The listing builds one solid part. Answer for the finished solid, in the listing's coordinates (mm). A direction names the side the tool comes from. Coordinates: 2 decimals unless noted, no trailing zeros. Write each loop counter-clockwise with the first axis right and the second up, starting at its lowest first coordinate (ties: lowest second). Pieces come first, ordered by that corner, then holes. Notation, with made-up numbers: M -19.75,8 L 33.25,8 A17 cw 33.25,24 Z; hole C 47,36 d1. An arc over 180 degrees is marked long. Write item = value, one per line. Start each with the question number.
```python
from build123d import *

# Parameters (mm, degrees)
SKETCH_1_R          = 1
EXTRUDE_1_DEPTH     = 7
SKETCH_2_R          = 3.75
EXTRUDE_2_DEPTH     = 1
SKETCH_3_W          = 8.378804874
SKETCH_3_H          = 1
CUT_EXTRUDE_1_DEPTH = 0.5


with BuildPart() as part:
    # 草图1 → 拉伸1 (new body)
    with BuildSketch(Plane(origin=(0, 0, 0), x_dir=(1, 0, 0), z_dir=(0, 1, 0))):
        with Locations(Location((0, 0, 0), (0, 0, 270))):
            Circle(SKETCH_1_R)
    extrude(amount=EXTRUDE_1_DEPTH)

    # 草图2 → 拉伸2 (add)
    with BuildSketch(Plane(origin=(0, 7, 0), x_dir=(-1, 0, 0), z_dir=(0, 1, 0))):
        with Locations(Location((0, 0, 0), (0, 0, 90))):
            Circle(SKETCH_2_R)
    extrude(amount=EXTRUDE_2_DEPTH)

    # 草图3 → 切除-拉伸1 (cut)
    with BuildSketch(Plane(origin=(0, 8, 0), x_dir=(-1, 0, 0), z_dir=(0, 1, 0))):
        Rectangle(SKETCH_3_W, SKETCH_3_H)
    extrude(amount=-CUT_EXTRUDE_1_DEPTH, mode=Mode.SUBTRACT)


solid = part.part
```
1. The part is cut by section C-C, the plane y = 3.75. Write down the section's boundary in (x, z), and give its area (3 significant figures).
2. Straight lines are drawn through the part: L1, parallel to Y at x = 3, z = 1; L2, parallel to Z at x = -0.25, y = 4.25; L3, parallel to X at y = 0.5, z = -0.5. For each, find the intervals that lie inside material, in ascending order. Write a range as [from, to].
3. For a pull along Z with two mould halves and no side action, classify faces 1 (the face through (0, 7.5, 0)), 2 (the face through (0, 8, 2)), 3 (the face through (-1, 3, 0)) as pulls with the +Z half, pulls with the -Z half, needs draft (parallel to the pull), parting line crosses it, or undercut.
4. Each of these flat-tipped pins is pushed along its axis until it touches: pin 1 (4 mm diameter, centred on y = 3.5, z = 0, fed in from +X); pin 2 (0.8 mm diameter, centred on x = -1.5, z = 0, fed in from +Y); pin 3 (1 mm diameter, centred on x = 0.5, y = 3, fed in from -Z). Where does it stop, or does it pass through?
5. For faces 4 (the face through (0, 0, 0)), 5 (the face through (-1, 7, 1)), determine the directions among +Z, -Z, +X, -X, +Y, -Y from which every point of the face is accessible in a straight line to the end or side of a thin tool.
6. The part is cut by section A-A, the plane z = 0. Write down the section's boundary in (x, y).
7. The part is cut by section B-B, the plane x = 0. Write down the section's boundary in (y, z).
8. The part is cut by section D-D, the plane x = -3. Write down the section's boundary in (y, z).
Solution:
q1.outline = C 0,0 d2
q1.area = 3.14 mm^2
q2.L1 = [7, 8]
q2.L2 = [-0.97, 0.97]
q2.L3 = [-0.87, 0.87]
q3.face_1 = undercut
q3.face_2 = needs draft
q3.face_3 = parting line crosses it
q4.pin_1 = 1
q4.pin_2 = 7.5
q4.pin_3 = -1
q5.face_4 = +Z, -Z, +X, -X, -Y
q5.face_5 = -Y
q6.outline = M -3.75,7 L -1,7 L -1,0 L 1,0 L 1,7 L 3.75,7 L 3.75,7.5 L -3.75,7.5 Z
q7.outline = M 0,-1 L 7,-1 L 7,-3.75 L 8,-3.75 L 8,-0.5 L 7.5,-0.5 L 7.5,0.5 L 8,0.5 L 8,3.75 L 7,3.75 L 7,1 L 0,1 Z
q8.outline = M 7,-2.25 L 8,-2.25 L 8,-0.5 L 7.5,-0.5 L 7.5,0.5 L 8,0.5 L 8,2.25 L 7,2.25 Z
